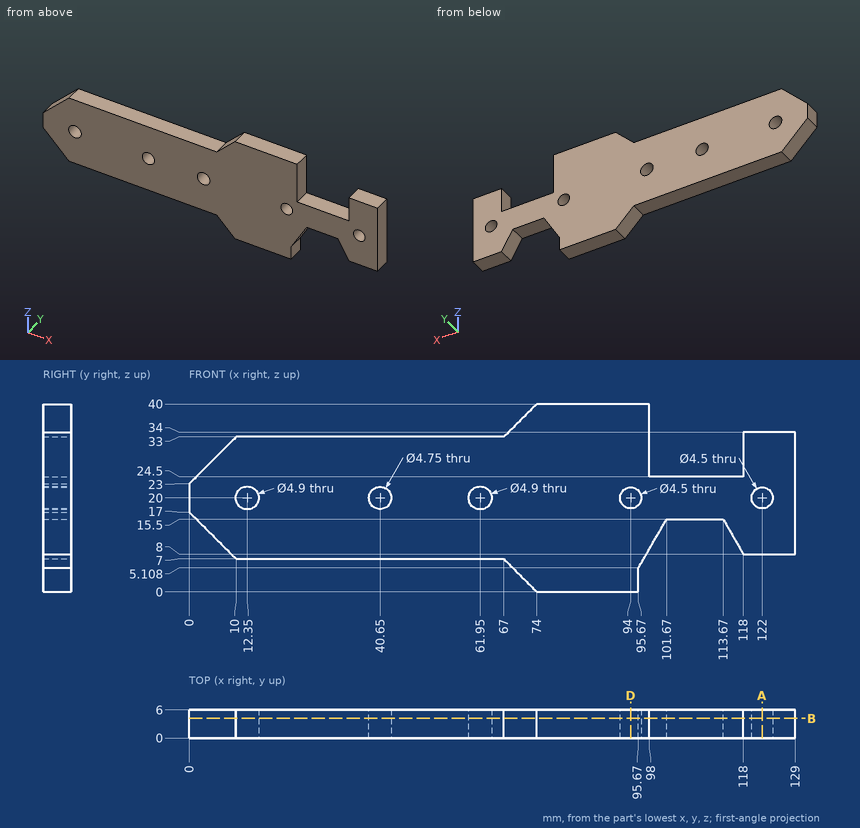
Source: three-view drawing plus pictorial views. Frame: mm from the lowest corner of the part. Give positions to 0.01 mm unless a question says otherwise; leave off trailing zeros. Loops run counter-clockwise (first coordinate to the right, second up) from the corner with the lowest first, then second, coordinate; pieces in that order, holes last. Notation, with made-up numbers: (89, -29) -> (130, -29) arc R17 cw to (130, 3) -> close; hole circle Ø3 at (19.5, 85.5). An arc over 180 degrees is marked (long way). Put each result on its own line as item: value. Start each with the question number.
1) Contact query for flat-ended pins moving along their axis: P1, Ø1.8, axis at x = 38.5, y = 3, coming from the +Z side; P2, Ø1, axis at x = 26.5, y = 1, coming from the -Z side; P3, Ø1.8, axis at x = 123.5, y = 2.5, coming from the +Z side. Output: stop coordinate, or through.
2) Cut plane A-A (x = 122). Return loops of the section in (y, z), then the cut area to 3 significant figures.
3) Material intervals for probe 1 along Z at (x, y) = (122, 4.3); probe 2 along Z at (x, y) = (94, 4.7); probe 3 along X at (y, z) = (2.2, 30), sorted ascending.
4) Cut plane D-D (x = 94). Return loops of the section in (y, z), then the cut area to 3 significant figures.
5) Cut plane B-B (y = 4.2). State how many separate pieces and enclosed holes the cut face has, then the cut area to 3 significant figures.
Results are:
1. P1: stops at z = 33
1. P2: stops at z = 7
1. P3: stops at z = 34
2. outline: (0, 8) -> (6, 8) -> (6, 17.75) -> (0, 17.75) -> close; (0, 22.25) -> (6, 22.25) -> (6, 34) -> (0, 34) -> close
2. area: 129 mm2
3. probe 1: z = 8 to 17.75, 22.25 to 34
3. probe 2: z = 0 to 17.75, 22.25 to 40
3. probe 3: x = 7 to 98, 118 to 129
4. outline: (0, 0) -> (6, 0) -> (6, 17.75) -> (0, 17.75) -> close; (0, 22.25) -> (6, 22.25) -> (6, 40) -> (0, 40) -> close
4. area: 213 mm2
5. separate pieces: 1
5. enclosed holes: 5
5. area: 3,220 mm2
